```python
from build123d import *

# Parameters (mm, degrees)
SKETCH1_R           = 2.6035
BOSS_EXTRUDE1_DEPTH = 558.8


with BuildPart() as part:
    # Sketch1 → Boss-Extrude1 (new body)
    with BuildSketch(Plane(origin=(0, 0, -558.8), x_dir=(-1, 0, 0), z_dir=(0, 0, -1))):
        with BuildLine():
            Line((12.699999967, -9.5504), (12.699999967, -6.3246))
            ThreePointArc((12.699999967, -6.3246), (12.191999967, -5.8166), (12.699999967, -5.3086))
            Line((12.699999967, -5.3086), (12.699999967, 5.3086))
            ThreePointArc((12.699999967, 5.3086), (12.191999967, 5.8166), (12.699999967, 6.3246))
            Line((12.699999967, 6.3246), (12.699999967, 9.550399967))
            ThreePointArc((12.699999967, 9.550399967), (12.191999934, 10.058400016), (12.699999999, 10.566400033))
            ThreePointArc((12.699999999, 10.566400033), (12.082677404, 12.082677438), (10.566399999, 12.700000033))
            ThreePointArc((10.566399999, 12.700000033), (10.058400007, 12.192000016), (9.550399999, 12.700000016))
            Line((9.550399999, 12.700000016), (6.324599999, 12.700000016))
            ThreePointArc((6.324599999, 12.700000016), (5.816599999, 12.192000016), (5.308599999, 12.700000016))
            Line((5.308599999, 12.700000016), (4.302307888, 12.700000016))
            ThreePointArc((4.302307888, 12.700000016), (3.197407888, 11.595100016), (4.302307888, 10.490200016))
            Line((4.302307888, 10.490200016), (6.474794464, 10.490200016))
            ThreePointArc((6.474794464, 10.490200016), (7.413456072, 9.863006381), (7.193214956, 8.755779521))
            Line((7.193214956, 8.755779521), (3.875871421, 5.438435986))
            ThreePointArc((3.875871421, 5.438435986), (2.845827288, 4.7501825), (1.63080739, 4.508500016))
            Line((1.63080739, 4.508500016), (-1.630807376, 4.508500016))
            ThreePointArc((-1.630807376, 4.508500016), (-2.845827273, 4.7501825), (-3.875871406, 5.438435986))
            Line((-3.875871406, 5.438435986), (-7.193214947, 8.755779526))
            ThreePointArc((-7.193214947, 8.755779526), (-7.413456062, 9.863006383), (-6.474794457, 10.490200016))
            Line((-6.474794457, 10.490200016), (-4.302307919, 10.490200016))
            ThreePointArc((-4.302307919, 10.490200016), (-3.197407919, 11.595100016), (-4.302307919, 12.700000016))
            Line((-4.302307919, 12.700000016), (-5.308600001, 12.700000016))
            ThreePointArc((-5.308600001, 12.700000016), (-5.816600001, 12.192000016), (-6.324600001, 12.700000016))
            Line((-6.324600001, 12.700000016), (-9.550400001, 12.700000016))
            ThreePointArc((-9.550400001, 12.700000016), (-10.058400001, 12.192000016), (-10.566400001, 12.700000016))
            ThreePointArc((-10.566400001, 12.700000016), (-12.082677418, 12.082677417), (-12.700000017, 10.5664))
            ThreePointArc((-12.700000017, 10.5664), (-12.192, 10.058400008), (-12.7, 9.5504))
            Line((-12.7, 9.5504), (-12.7, 6.3246))
            ThreePointArc((-12.7, 6.3246), (-12.192, 5.8166), (-12.7, 5.3086))
            Line((-12.7, 5.3086), (-12.7, 4.302307889))
            ThreePointArc((-12.7, 4.302307889), (-11.5951, 3.197407889), (-10.4902, 4.302307889))
            Line((-10.4902, 4.302307889), (-10.4902, 6.474794456))
            ThreePointArc((-10.4902, 6.474794456), (-9.863006367, 7.413456061), (-8.75577951, 7.193214945))
            Line((-8.75577951, 7.193214945), (-5.43843597, 3.875871405))
            ThreePointArc((-5.43843597, 3.875871405), (-4.750182484, 2.845827272), (-4.5085, 1.630807374))
            Line((-4.5085, 1.630807374), (-4.5085, -1.630807374))
            ThreePointArc((-4.5085, -1.630807374), (-4.750182484, -2.845827272), (-5.43843597, -3.875871405))
            Line((-5.43843597, -3.875871405), (-8.75577951, -7.193214945))
            ThreePointArc((-8.75577951, -7.193214945), (-9.863006367, -7.413456061), (-10.4902, -6.474794456))
            Line((-10.4902, -6.474794456), (-10.4902, -4.302307918))
            ThreePointArc((-10.4902, -4.302307918), (-11.5951, -3.197407918), (-12.7, -4.302307918))
            Line((-12.7, -4.302307918), (-12.7, -5.3086))
            ThreePointArc((-12.7, -5.3086), (-12.192, -5.8166), (-12.7, -6.3246))
            Line((-12.7, -6.3246), (-12.7, -9.5504))
            ThreePointArc((-12.7, -9.5504), (-12.192, -10.058400008), (-12.700000017, -10.5664))
            ThreePointArc((-12.700000017, -10.5664), (-12.082677422, -12.082677406), (-10.566400017, -12.7))
            ThreePointArc((-10.566400017, -12.7), (-10.058400017, -12.192), (-9.550400017, -12.7))
            Line((-9.550400017, -12.7), (-6.324600017, -12.7))
            ThreePointArc((-6.324600017, -12.7), (-5.816600017, -12.192), (-5.308600017, -12.7))
            Line((-5.308600017, -12.7), (5.308599983, -12.7))
            ThreePointArc((5.308599983, -12.7), (5.816599983, -12.192), (6.324599983, -12.7))
            Line((6.324599983, -12.7), (9.550399983, -12.7))
            ThreePointArc((9.550399983, -12.7), (10.058399983, -12.192), (10.566399983, -12.7))
            ThreePointArc((10.566399983, -12.7), (12.082677389, -12.082677406), (12.699999983, -10.5664))
            ThreePointArc((12.699999983, -10.5664), (12.191999967, -10.058400008), (12.699999967, -9.5504))
        make_face()
        Circle(SKETCH1_R, mode=Mode.SUBTRACT)
        with BuildLine():
            Line((3.875871405, -5.43843597), (7.13192049, -8.694485055))
            ThreePointArc((7.13192049, -8.694485055), (7.35441848, -9.056211656), (7.4295, -9.4742))
            ThreePointArc((7.4295, -9.4742), (7.13192049, -10.19262049), (6.4135, -10.4902))
            Line((6.4135, -10.4902), (-6.4135, -10.4902))
            ThreePointArc((-6.4135, -10.4902), (-7.13192049, -10.19262049), (-7.4295, -9.4742))
            ThreePointArc((-7.4295, -9.4742), (-7.35441848, -9.056211656), (-7.13192049, -8.694485055))
            Line((-7.13192049, -8.694485055), (-3.875871405, -5.43843597))
            ThreePointArc((-3.875871405, -5.43843597), (-2.845827272, -4.750182484), (-1.630807374, -4.5085))
            Line((-1.630807374, -4.5085), (1.630807374, -4.5085))
            ThreePointArc((1.630807374, -4.5085), (2.845827272, -4.750182484), (3.875871405, -5.43843597))
        make_face(mode=Mode.SUBTRACT)
        with BuildLine():
            Line((10.490199999, 6.4135), (10.490199999, -6.413499984))
            ThreePointArc((10.490199999, -6.413499984), (10.192620488, -7.131920474), (9.474199999, -7.429499984))
            ThreePointArc((9.474199999, -7.429499984), (9.056211655, -7.354418464), (8.694485053, -7.131920474))
            Line((8.694485053, -7.131920474), (5.438435968, -3.875871389))
            ThreePointArc((5.438435968, -3.875871389), (4.750182483, -2.845827256), (4.508499999, -1.630807359))
            Line((4.508499999, -1.630807359), (4.508499999, 1.630807373))
            ThreePointArc((4.508499999, 1.630807373), (4.750182483, 2.845827271), (5.438435968, 3.875871403))
            Line((5.438435968, 3.875871403), (8.694485055, 7.13192049))
            ThreePointArc((8.694485055, 7.13192049), (9.056211656, 7.35441848), (9.4742, 7.4295))
            ThreePointArc((9.4742, 7.4295), (10.192620489, 7.131920489), (10.490199999, 6.4135))
        make_face(mode=Mode.SUBTRACT)
    extrude(amount=-BOSS_EXTRUDE1_DEPTH)


solid = part.part
```
Part model, mm, in its own coordinate system. Round coordinates to 2 decimals unless told otherwise and drop trailing zeros. Put each result on its own line as item: value. Start each with the question number.
1. Slice it at A-A on z = -105. State how many separate pieces and enclosed holes the cut face has, then the cut area to 3 significant figures.
2. Drop flat-ended pins along their axis: pin 1 (4.5 mm diameter, centred on x = 0, y = 0, fed in from -Z); pin 2 (3.5 mm diameter, centred on y = -0.5, z = -284, fed in from +X); pin 3 (3.5 mm diameter, centred on x = -0.5, z = -373.5, fed in from +Y). Give the stop position or say it passes through.
3. Drill centre lines: probe 1 along X at (y, z) = (-5.5, -367); probe 2 along Y at (x, z) = (0, -366.5); probe 3 along Y at (x, z) = (6.25, -199) (3 decimals). Where is each one in solid material? Low to high. Write a range as [from, to].
4. Two-plate mould, pull along X, no slides. Class faces 1 (the face through (0, -10.49, -283)), 2 (the face through (-10.49, 0, -283)), 3 (the face through (-3, 0, -558.8)), 4 (the face through (-12.7, 0, -283)): +X half, -X half, draft (parallel to the pull), parting line (faces both ways), or undercut.
Findings:
1. separate pieces: 1
1. enclosed holes: 3
1. area: 311 mm2
2. pin 1: through
2. pin 2: x = 4.57
2. pin 3: y = 4.57
3. probe 1: [-12.3, -10.49], [-7.06, -3.94], [3.94, 7.06], [10.49, 12.3]
3. probe 2: [-12.7, -10.49], [-4.51, -2.6], [2.6, 4.51]
3. probe 3: [-12.435, -10.49], [-7.813, -4.687], [4.687, 7.813], [10.49, 12.435]
4. face 1: undercut
4. face 2: undercut
4. face 3: draft
4. face 4: -X half
